```python
from build123d import *

# Parameters (mm, degrees)
F0_R     = 4
F1_DEPTH = 10
F3_COUNT = 3
F3_ANGLE = 240
F4_R     = 23.0054
F5_DEPTH = 25


with BuildPart() as f1:
    # F0 (on Front) → F1 (new body)
    with BuildSketch(Plane.XZ):
        with BuildLine():
            Line((10, 0), (-10, 0))
            Line((-10, 0), (-10, -290))
            ThreePointArc((-10, -290), (-7.071068, -297.071068), (0, -300))
            ThreePointArc((0, -300), (7.071068, -297.071068), (10, -290))
            Line((10, -290), (10, 0))
        make_face()
        with Locations((0, -290)):
            Circle(F0_R, mode=Mode.SUBTRACT)
    extrude(amount=F1_DEPTH)



with BuildPart() as f3_1:
    # F3: instance of F1
    add(f1.part.rotate(Axis((0, -33.912361, 0), (0, -1, 0)), 1 * F3_ANGLE / (F3_COUNT - 1)))


with BuildPart() as f3_2:
    # F3: instance of F1
    add(f1.part.rotate(Axis((0, -33.912361, 0), (0, -1, 0)), 2 * F3_ANGLE / (F3_COUNT - 1)))


with BuildPart() as f1_1:
    add(f1.part)

    add(f3_1.part)  # F5 merges F3_1

    add(f3_2.part)  # F5 merges F3_2
    # F4 (on face) → F5 (join)
    with BuildSketch(Plane(origin=(0, 0, 0), x_dir=(-1, 0, 0), z_dir=(0, 1, 0))):
        Circle(F4_R)
    extrude(amount=F5_DEPTH)


solid = f1_1.part
```
CAD build for the part. Positions are in the model's coordinates, mm. A direction names the side the tool comes from. Coordinates: 2 decimals unless noted, no trailing zeros. Order: outer loops, then holes, each group sorted by start corner. A loop starts at its lowest first (then second) coordinate and runs counter-clockwise, first axis right, second up. Notation, with made-up numbers: M 86.25,-30.75 L 108.25,-30.75 A25 cw 108.25,8.25 Z; hole C 25.25,45.25 d1. An arc over 180 degrees is marked long. Write each question's results on one line, items separated by ' | '. Start each with the question number.
Q1. Cut at D-D (x = -51). List the corners of the cut face in (y, z).
Q2. Pull direction X, two halves, no side cores. Call faces 5 (the flat face through (0, 0, 19)), 6 (the cylindrical face through (-21.943, 12.325, 6.91)), 7 (the flat face through (4, -10, 1)): +X half, -X half, draft (parallel to the pull), parting line (faces both ways), or undercut.
Q3. Cut at B-B (z = -182.5). List the corners of the cut face in (x, y), then the cut area to 3 significant figures.
Q4. Flat gauge pins, fed straight in: P1, Ø8, axis at y = -3, z = -203, coming from the +X side; P2, Ø2, axis at y = 8, z = -18.5, coming from the -X side; P3, Ø5, axis at y = -3, z = -165.5, coming from the -X side. Where does each tip first touch, or does it go through?
Q5. Drill centre lines: probe 1 along X at (y, z) = (-2, -290); probe 2 along Z at (x, y) = (0, -3); probe 3 along Z at (x, y) = (-2, 13). Where is each one in solid material? Low to high. Write a range as from..to.
Q6. Cut at A-A (z = 64.5). List the corners of the cut face in (x, y).
Q7. Which spindle directions (+Z, -Z, +X, -X, +Y, -Y) get a long thin tool onto all of the face, cutting with end or side? Do faces 1 (the flat face through (1, 0, -159)), 2 (the flat face through (0, 25, 0)), 3 (the flat face through (-16, 0, -9)), 4 (the flat face through (17, 0, -9)). Say none if no direction does.
Q8. Cut at C-C (y = 18). List the corners of the cut face in (x, z).
Found:
1) outline: M -10,17.9 L 0,17.9 L 0,40.99 L -10,40.99 Z
2) face 5: undercut | face 6: parting line | face 7: draft
3) outline: M -10,-10 L 10,-10 L 10,0 L -10,0 Z | area: 200 mm²
4) P1: x = 10 | P2: x = -14.93 | P3: x = -10
5) probe 1: -10..-4, 4..10 | probe 2: -300..-294, -286..11.55 | probe 3: -22.92..22.92
6) outline: M -131.72,-10 L -91.72,-10 L -91.72,0 L -131.72,0 Z; M 91.72,-10 L 131.72,-10 L 131.72,0 L 91.72,0 Z
7) face 1: -Z, +X, -X, +Y | face 2: +Z, -Z, +X, -X, +Y | face 3: -Z, -X, -Y | face 4: -Z, +X, -Y
8) outline: C 0,0 d46.01
